```python
from build123d import *

# Parameters (mm, degrees)
SKETCH1_W           = 537
SKETCH1_H           = 80
BOSS_EXTRUDE1_DEPTH = 3
CAVITY1_START       = 37
CAVITY1_OUTLINE_W   = 15.5
CAVITY1_OUTLINE_H   = 3
CAVITY1_OUTLINE_W_2 = 9.5
CAVITY1_DEPTH       = 3


# Read off the part's stored shape, not the designer's step: Cavity1
with BuildPart() as part:
    # Sketch1 → Boss-Extrude1 (new body)
    with BuildSketch(Plane.XY):
        Rectangle(SKETCH1_W, SKETCH1_H)
    extrude(amount=BOSS_EXTRUDE1_DEPTH)

    # Cavity1 outline → Cavity1 (cut)
    with BuildSketch(Plane(origin=(0, 0, 0), x_dir=(1, 0, 0), z_dir=(0, 1, 0)).offset(CAVITY1_START)):
        with Locations((-236.25, -1.5)):
            Rectangle(CAVITY1_OUTLINE_W, CAVITY1_OUTLINE_H)
        with Locations((-263.75, -1.5)):
            Rectangle(CAVITY1_OUTLINE_W_2, CAVITY1_OUTLINE_H)
        with Locations((-205.75, -1.5)):
            Rectangle(CAVITY1_OUTLINE_W, CAVITY1_OUTLINE_H)
        with Locations((-175.25, -1.5)):
            Rectangle(CAVITY1_OUTLINE_W, CAVITY1_OUTLINE_H)
        with Locations((-144.75, -1.5)):
            Rectangle(CAVITY1_OUTLINE_W, CAVITY1_OUTLINE_H)
        with Locations((-114.25, -1.5)):
            Rectangle(CAVITY1_OUTLINE_W, CAVITY1_OUTLINE_H)
        with Locations((-83.75, -1.5)):
            Rectangle(CAVITY1_OUTLINE_W, CAVITY1_OUTLINE_H)
        with Locations((-53.25, -1.5)):
            Rectangle(CAVITY1_OUTLINE_W, CAVITY1_OUTLINE_H)
        with Locations((-22.75, -1.5)):
            Rectangle(CAVITY1_OUTLINE_W, CAVITY1_OUTLINE_H)
        with Locations((22.75, -1.5)):
            Rectangle(CAVITY1_OUTLINE_W, CAVITY1_OUTLINE_H)
        with Locations((53.25, -1.5)):
            Rectangle(CAVITY1_OUTLINE_W, CAVITY1_OUTLINE_H)
        with Locations((83.75, -1.5)):
            Rectangle(CAVITY1_OUTLINE_W, CAVITY1_OUTLINE_H)
        with Locations((114.25, -1.5)):
            Rectangle(CAVITY1_OUTLINE_W, CAVITY1_OUTLINE_H)
        with Locations((144.75, -1.5)):
            Rectangle(CAVITY1_OUTLINE_W, CAVITY1_OUTLINE_H)
        with Locations((175.25, -1.5)):
            Rectangle(CAVITY1_OUTLINE_W, CAVITY1_OUTLINE_H)
        with Locations((205.75, -1.5)):
            Rectangle(CAVITY1_OUTLINE_W, CAVITY1_OUTLINE_H)
        with Locations((236.25, -1.5)):
            Rectangle(CAVITY1_OUTLINE_W, CAVITY1_OUTLINE_H)
        with Locations((263.75, -1.5)):
            Rectangle(CAVITY1_OUTLINE_W_2, CAVITY1_OUTLINE_H)
    extrude(amount=CAVITY1_DEPTH, mode=Mode.SUBTRACT)


solid = part.part
```
Build history of the part. All positions in model axes, mm. Give positions to 0.01 mm unless a question says otherwise; leave off trailing zeros. Loops run counter-clockwise (first coordinate to the right, second up) from the corner with the lowest first, then second, coordinate; pieces in that order, holes last. Notation, with made-up numbers: (-0.5, 34.5) -> (30.5, 34.5) arc R17 cw to (30.5, 55.5) -> close; hole circle Ø6 at (53.5, 75). An arc over 180 degrees is marked (long way). One line per question, with ' | ' between items. Start each with the question number.
1) Pin check, flat tips, straight feed: pin 1 (1.5 mm diameter, centred on x = -239.5, z = 1.5, fed in from +Y); pin 2 (0.9 mm diameter, centred on y = 39, z = 1, fed in from +X); pin 3 (1.5 mm diameter, centred on y = 39, z = 1, fed in from -X). Stop position of each tip, or through.
2) Probe L1, parallel to Y at x = -48, z = 2.35. List the from-to ranges inside material, lowest first.
3) Cut at A-A (x = 86.5). Give the cut face in (y, z).
Return value:
1) pin 1: y = 37 | pin 2: x = 259 | pin 3: x = -259
2) L1: -40 to 37
3) outline: (-40, 0) -> (37, 0) -> (37, 3) -> (-40, 3) -> close
